For this review, take the finished solid that the model builds, in its own axes (mm). Face numbers are marked on the shaded views. Coordinates: 2 decimals unless noted, no trailing zeros. Write each loop counter-clockwise with the first axis right and the second up, starting at its lowest first coordinate (ties: lowest second). Pieces come first, ordered by that corner, then holes.
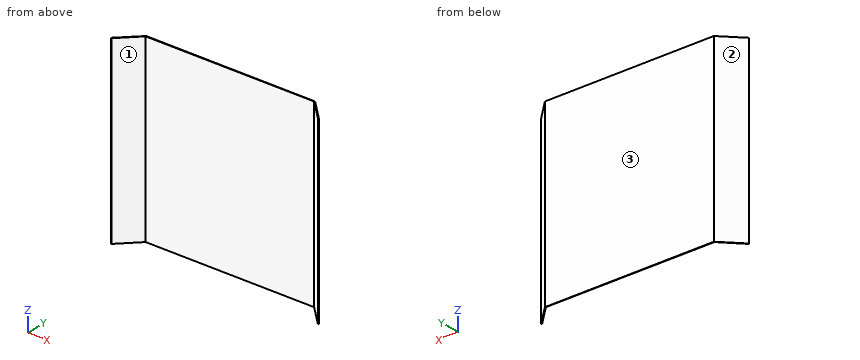
Autodesk Inventor part; units mm, degrees
ref_plane "YZ Plane" through (0, 0, 0) normal (1, 0, 0) x (0, 1, 0)
ref_plane "XZ Plane" through (0, 0, 0) normal (0, 1, 0) x (-1, 0, 0)
ref_plane "XY Plane" through (0, 0, 0) normal (0, 0, 1) x (1, 0, 0)
sketch "Sketch1" plane through (0, 0, 0) normal (0, 0, 1) x (1, 0, 0)
  line L0 (0, 0) -> (53.8815, 53.8815)
  line L1 (0, 0) -> (76.2, 0) construction
  line L2 (0, 0) -> (1.4368, -1.4368)
  line L3 (53.8815, 53.8815) -> (523.7815, 53.8815) construction
  line L4 (523.7815, 53.8815) -> (577.6409, -0.0222)
  line L5 (577.6409, -0.0222) -> (576.2034, -1.4585)
  line L6 (523.7815, 53.8815) -> (525.8135, 53.8815) construction
  line L7 (522.3441, 52.4453) -> (576.2034, -1.4585)
  line L8 (53.8815, 51.8495) -> (1.4368, -1.4368)
  line L9 (53.8815, 51.8495) -> (522.3441, 52.4453)
  line L10 (53.8815, 53.8815) -> (523.7815, 53.8815)
  dimension "d0" = 76.2
  dimension "d1" = 45
  dimension "d2" = 2.032
  dimension "d5" = 76.2
  dimension "d6" = 2.032
  dimension "d7" = 2.032
  dimension "d9" = 2.032
extrude "Extrusion1" add sketch "Sketch1" along normal blind 508
properties part number "LoadSlide" material "Polycarbonate, Clear"
Q1. Add section C-C (y = 9). State the section outline as (x, z) points.
Ans:
outline: (9, 0) - (11.71, 0) - (11.71, 508) - (9, 508) - close; (565.75, 0) - (568.63, 0) - (568.63, 508) - (565.75, 508) - close
Q2. Add section D-D (x = 330). State the section outline as (y, z) points, then the cut area to 3 significant figures.
Ans:
outline: (52.2, 0) - (53.88, 0) - (53.88, 508) - (52.2, 508) - close
area: 854 mm2
Q3. Clearance check with flat-ended pins moving along their axes: pin 1 Ø3 at (y, z) = (9.5, 156.5) entering from +X; pin 2 Ø4 at (y, z) = (12, 435.5) entering from +X; pin 3 Ø1 at (y, z) = (41, 264.5) entering from -X. State where each tip first meets the part, or that it passes through.
Ans:
pin 1: stops at x = 569.63
pin 2: stops at x = 567.63
pin 3: stops at x = 40.5
Q4. Add section B-B (z = 346.5). State the section outline as (x, y) points.
Ans:
outline: (0, 0) - (1.44, -1.44) - (53.88, 51.85) - (522.34, 52.45) - (576.2, -1.46) - (577.64, -0.02) - (523.78, 53.88) - (53.88, 53.88) - close
Q5. For probe 1 along Y at (x, z) = (105.5, 461); probe 2 along X at (y, z) = (40.5, 372); probe 3 along X at (y, z) = (44.5, 223), list the stretches that pass through material, from the lowest coordinate up.
Ans:
probe 1: y = 51.92 to 53.88
probe 2: x = 40.5 to 42.71, 534.28 to 537.15
probe 3: x = 44.5 to 46.65, 530.28 to 533.16
Q6. Draft analysis for pull direction X (two halves, no side actions). For the marked faces 1, 2 and 3, state which applies: +X half, -X half, draft (parallel to the pull), parting line (faces both ways), or undercut.
Ans:
face 1: undercut
face 2: -X half
face 3: draft
Q7. Add section A-A (y = 38). State the section outline as (x, z) points.
Ans:
outline: (38, 0) - (40.25, 0) - (40.25, 508) - (38, 508) - close; (536.78, 0) - (539.65, 0) - (539.65, 508) - (536.78, 508) - close
